Source: three-view drawing plus pictorial views. Frame: mm from the lowest corner of the part. A direction names the side the tool comes from. Coordinates: 2 decimals unless noted, no trailing zeros. Loops run counter-clockwise (first coordinate to the right, second up) from the corner with the lowest first, then second, coordinate; pieces in that order, holes last. Notation, with made-up numbers: (79.5, 79.5) - (137.5, 79.5) arc R21 ccw to (137.5, 112.5) - close; hole circle Ø8 at (-25, 23). An arc over 180 degrees is marked (long way). Return JSON: item names as keys, results as strings.
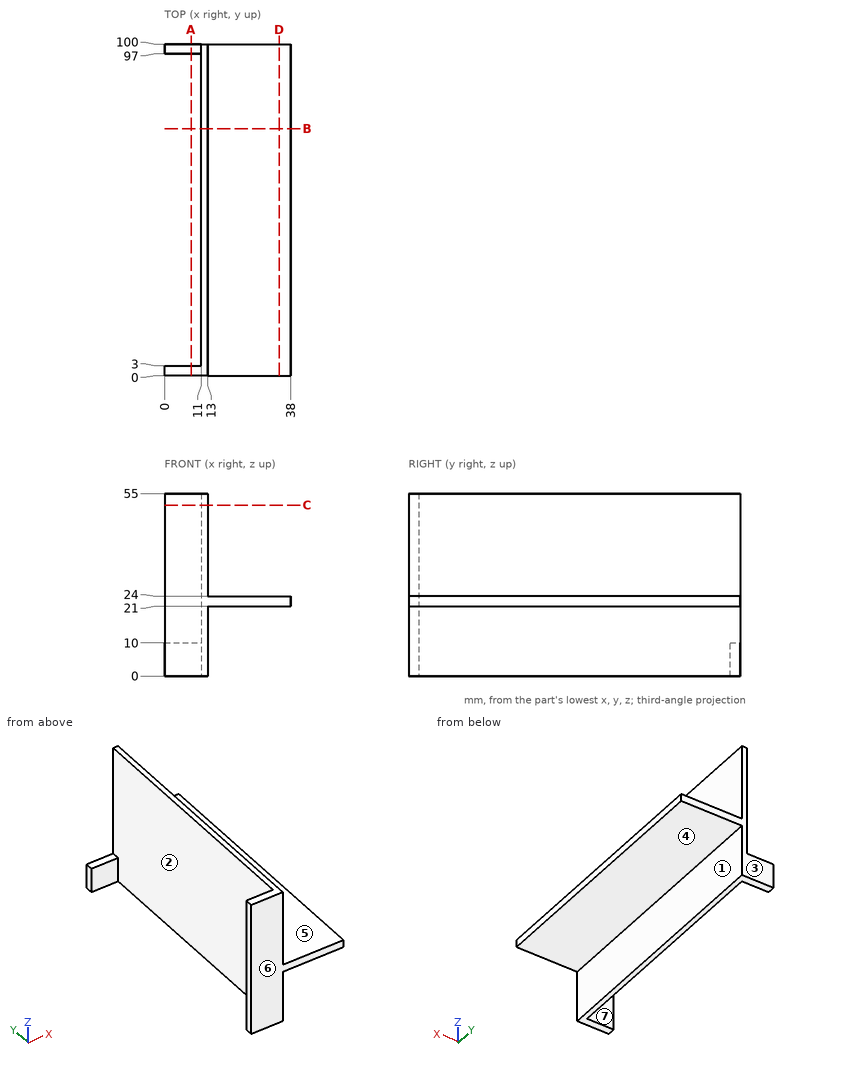
Item 1: Section query B-B, the plane y = 74.5. Return loops of the section in (x, z), and give its area (3 significant figures).
Worked out:
{"outline": "(11, 0) - (13, 0) - (13, 21) - (38, 21) - (38, 24) - (13, 24) - (13, 55) - (11, 55) - close", "area": "185 mm^2"}
Item 2: Reachability of the marked faces 4, 5, 6 and 7 from +Z, -Z, +X, -X, +Y, -Y: full face, straight path, thin tool, end or side. Return the list, or none.
Worked out:
{"face 4": "-Z, +X, +Y, -Y", "face 5": "+Z, +X, +Y, -Y", "face 6": "+Z, -Z, +X, -X, -Y", "face 7": "+Z, -Z, -X"}
Item 3: Ray query, probe 1 along Y at (x, z) = (4.5, 6); probe 2 along X at (y, z) = (5, 23); probe 3 along Y at (x, z) = (8, 42). Return the intervals inside material, ascending. Write a range as from..to.
Worked out:
{"probe 1": "0..3, 97..100", "probe 2": "11..38", "probe 3": "0..3"}
Item 4: Section query A-A, the plane x = 8. Return loops of the section in (y, z), and give its area (3 significant figures).
Worked out:
{"outline": "(0, 0) - (3, 0) - (3, 55) - (0, 55) - close; (97, 0) - (100, 0) - (100, 10) - (97, 10) - close", "area": "195 mm^2"}
Item 5: Section query C-C, the plane z = 51.5. Return loops of the section in (x, y), and give its area (3 significant figures).
Worked out:
{"outline": "(0, 0) - (13, 0) - (13, 100) - (11, 100) - (11, 3) - (0, 3) - close", "area": "233 mm^2"}
Item 6: Mould query, pull axis Y, two halves, no side actions, for the marked faces 1, 2 and 3. Classes: +Y half, -Y half, draft (parallel to the pull), parting line (faces both ways), or undercut.
Worked out:
{"face 1": "draft", "face 2": "undercut", "face 3": "+Y half"}
Item 7: Section query D-D, the plane x = 34.5. Return loops of the section in (y, z), and give its area (3 significant figures).
Worked out:
{"outline": "(0, 21) - (100, 21) - (100, 24) - (0, 24) - close", "area": "300 mm^2"}
Item 8: First-contact query: pin 1 Ø10.5 at (y, z) = (40.5, 13) entering from +X; pin 2 Ø5 at (x, y) = (30.5, 21.5) entering from +Z; pin 3 Ø8 at (y, z) = (34, 28) entering from -X. Flat tips, straight axial feed; report the tip coordinate or a pass-through.
Worked out:
{"pin 1": "x = 13", "pin 2": "z = 24", "pin 3": "x = 11"}
